Check sheet for the drawn part. Datum: minimum x, y, z corner. Units: mm. A direction names the side the tool comes from. Coordinates: 2 decimals unless noted, no trailing zeros. Order: outer loops, then holes, each group sorted by start corner. A loop starts at its lowest first (then second) coordinate and runs counter-clockwise, first axis right, second up.
Q1. Thickness scan on line 1 (Y direction, x = 5, z = 8.75); line 2 (Y direction, x = 4.25, z = 18); line 3 (X direction, y = 8, z = 13). Record the ranges inside material, lowest first.
Q2. Depth check by flat-ended pin: P1, Ø1, axis at x = 7.5, y = 31, coming from the -Z side; P2, Ø12, axis at y = 16.5, z = 4.5, coming from the -X side; P3, Ø8, axis at x = 10.5, y = 49, coming from the +Z side. Enter the tip coordinate at first touch or a pass-through.
Q3. Cross-section at B-B, the plane x = 5. Record the boundary of the cut face in (y, z).
Q4. Set-up check for the marked faces 1, 2 and 3: record each of +Z, -Z, +X, -X, +Y, -Y from which the full face is reachable in a straight line by a thin tool's end or side.
Q5. Cross-section at C-C, the plane y = 42.5. Record the boundary of the cut face in (x, z), and give its area (3 significant figures).
Q6. Cross-section at A-A, the plane z = 13. Record the boundary of the cut face in (x, y).
Q7. Cross-section at D-D, the plane x = 13. Record the boundary of the cut face in (y, z).
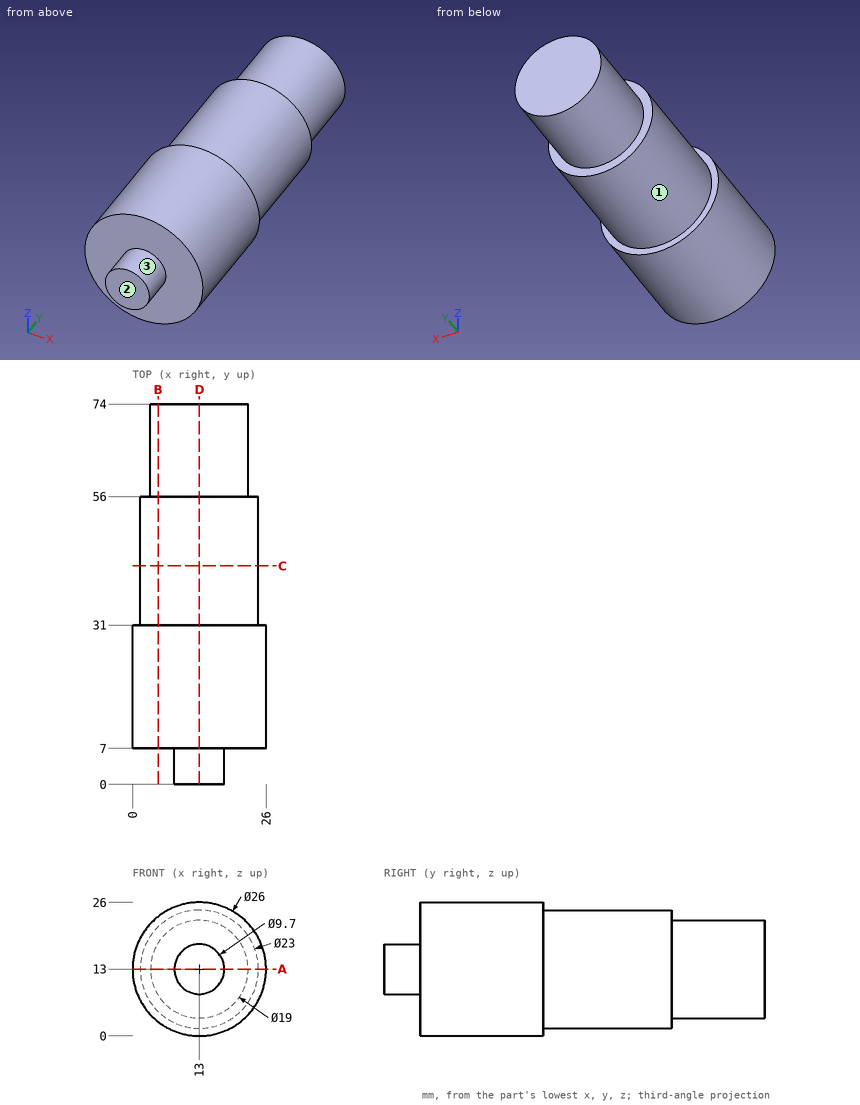
Check values:
1. line 1: y = 7 to 74
1. line 2: y = 7 to 56
1. line 3: x = 0 to 26
2. P1: stops at z = 1
2. P2: stops at x = 0.24
2. P3: stops at z = 24.5
3. outline: (7, 2.75) - (31, 2.75) - (31, 4.74) - (56, 4.74) - (56, 7.88) - (74, 7.88) - (74, 18.12) - (56, 18.12) - (56, 21.26) - (31, 21.26) - (31, 23.25) - (7, 23.25) - close
4. face 1: +Y
4. face 2: +Z, -Z, +X, -X, -Y
4. face 3: -Y
5. outline: circle Ø23 at (13, 13)
5. area: 415 mm2
6. outline: (0, 7) - (8.15, 7) - (8.15, 0) - (17.85, 0) - (17.85, 7) - (26, 7) - (26, 31) - (24.5, 31) - (24.5, 56) - (22.5, 56) - (22.5, 74) - (3.5, 74) - (3.5, 56) - (1.5, 56) - (1.5, 31) - (0, 31) - close
7. outline: (0, 8.15) - (7, 8.15) - (7, 0) - (31, 0) - (31, 1.5) - (56, 1.5) - (56, 3.5) - (74, 3.5) - (74, 22.5) - (56, 22.5) - (56, 24.5) - (31, 24.5) - (31, 26) - (7, 26) - (7, 17.85) - (0, 17.85) - close
